Build history of the part. All positions in model axes, mm. A direction names the side the tool comes from. Give positions to 0.01 mm unless a question says otherwise; leave off trailing zeros. Write each loop counter-clockwise with the first axis right and the second up, starting at its lowest first coordinate (ties: lowest second). Pieces come first, ordered by that corner, then holes. Notation, with made-up numbers: (8.25, -11.5) -> (37.25, -11.5) arc R32 ccw to (37.25, 24.5) -> close; hole circle Ø10 at (73.25, 50.5). An arc over 180 degrees is marked (long way). Put each result on its own line as item: value.
from build123d import *

# Parameters (mm, degrees)
BOSS_EXTRUDE1_DEPTH     = 8
BOSS_EXTRUDE2_DEPTH     = 8
SKETCH4_W               = 36.000000000000064
SKETCH4_H               = 30.000000000000057
BOSS_EXTRUDE3_DEPTH     = 8
SKETCH5_R               = 7.000000000000002
SKETCH5_R_2             = 5.000000000000002
BOSS_EXTRUDE4_DEPTH     = 10
CHAMFER1_SIZE           = 3
CUT_EXTRUDE1_REACH      = 260.278
CUT_EXTRUDE2_DEPTH      = 254.2099380250209
SKETCH8_W               = 17.000000000000007
SKETCH8_H               = 20.000000000000043
BOSS_EXTRUDE5_DEPTH     = 7
CUT_EXTRUDE3_DEPTH      = 0.75
CUT_EXTRUDE4_DEPTH      = 0.75
CUT_EXTRUDE5_DEPTH      = 254.2099381566107
CUT_EXTRUDE5_DEPTH_BACK = 254.2099381566107
CUT_EXTRUDE6_DEPTH      = 3
SKETCH14_W              = 9.999999998633207
SKETCH14_H              = 30.000000000000057
CUT_EXTRUDE7_DEPTH      = 3
CUT_EXTRUDE8_START      = -33
CUT_EXTRUDE8_DEPTH      = 30
SKETCH16_W              = 67.2347482813901
SKETCH16_H              = 36.897117956044724
CUT_EXTRUDE9_DEPTH      = 28.75


with BuildPart() as part:
    # Sketch2 → Boss-Extrude1 (new body)
    with BuildSketch(Plane.XY.offset(-8.000000000000261)):
        with BuildLine():
            Line((-25.76918534335193, 245.18029985394168), (-54.787386755608914, 245.18029985394168))
            Line((-54.787386755608914, 245.18029985394168), (-54.787386755608914, 215.18029985394165))
            Line((-54.787386755608914, 215.18029985394165), (-25.76918534335193, 215.18029985394165))
            ThreePointArc((-25.76918534335193, 215.18029985394165), (-10.7691853433519, 230.18029985394168), (-25.76918534335193, 245.18029985394168))
        make_face()
    extrude(amount=BOSS_EXTRUDE1_DEPTH)



with BuildPart() as body_2:
    # Sketch3 → Boss-Extrude2 (new body)
    with BuildSketch(Plane(origin=(4.616e-14, 1.89e-15, -28.000000000000256), x_dir=(-1, 0, -1.65e-15), z_dir=(1.65e-15, 7e-17, -1))):
        with BuildLine():
            Line((25.769185343351936, 215.18029985394165), (54.78738675560893, 215.18029985394165))
            Line((54.78738675560893, 215.18029985394165), (54.78738675560893, 245.18029985394168))
            Line((54.78738675560893, 245.18029985394168), (25.76918534335194, 245.18029985394168))
            ThreePointArc((25.76918534335194, 245.18029985394168), (10.769185343351939, 230.18029985394168), (25.769185343351936, 215.18029985394165))
        make_face()
    extrude(amount=BOSS_EXTRUDE2_DEPTH)


with BuildPart() as part_1:
    add(part.part)

    add(body_2.part)  # Boss-Extrude3 merges body 2
    # Sketch4 → Boss-Extrude3 (add)
    with BuildSketch(Plane.ZY.offset(54.787386755608914)):
        with Locations((-18.000000000000345, 230.18029985394168)):
            Rectangle(SKETCH4_W, SKETCH4_H)
    extrude(amount=BOSS_EXTRUDE3_DEPTH)

    # Sketch5 → Boss-Extrude4 (add)
    with BuildSketch(Plane.ZY.offset(62.78738675560891)):
        with Locations((-18.00000000000032, 230.18029985394168)):
            Circle(SKETCH5_R)
        with Locations((-18.00000000000032, 230.18029985394168)):
            Circle(SKETCH5_R_2, mode=Mode.SUBTRACT)
    extrude(amount=BOSS_EXTRUDE4_DEPTH)

    # Chamfer1
    chamfer1_edges = [part_1.edges().sort_by_distance(p)[0] for p in [
        (-62.78738675560891, 230.18029985394168, -25.00000000000032),
    ]]
    chamfer(chamfer1_edges, length=CHAMFER1_SIZE)

    # Cut-Extrude1: up to this face of the body (flat: up to its plane)
    cut_extrude1_end = Plane(part_1.part.faces().sort_by_distance((-38.272954764, 230.180299854, 0))[0])
    # Sketch6 → Cut-Extrude1 (cut, up to the picked face)
    with BuildSketch(Plane(origin=(0, 0, -36.00000000000038), x_dir=(-1, 0, 0), z_dir=(0, 0, -1)), mode=Mode.PRIVATE) as cut_extrude1_sk1:
        with BuildLine():
            Line((23.93206803626449, 232.05529985394165), (27.606302650439275, 232.05529985394165))
            ThreePointArc((27.606302650439275, 232.05529985394165), (28.39418534335189, 230.18029985394165), (27.606302650439247, 228.30529985394165))
            Line((27.606302650439247, 228.30529985394165), (23.932068036264518, 228.30529985394165))
            ThreePointArc((23.932068036264518, 228.30529985394165), (23.144185343351896, 230.18029985394165), (23.93206803626449, 232.05529985394165))
        make_face()
    cut_extrude1_tool1 = split(extrude(cut_extrude1_sk1.sketch, amount=-CUT_EXTRUDE1_REACH, mode=Mode.PRIVATE), bisect_by=cut_extrude1_end, keep=Keep.BOTH, mode=Mode.PRIVATE)
    add(cut_extrude1_tool1.solids().sort_by(Axis((-25.769185, 230.1803, -36), (0, 0, 1)))[0], mode=Mode.SUBTRACT)

    # Sketch7 → Cut-Extrude2 (cut, through all)
    with BuildSketch(Plane.ZY.offset(62.78738675560891)):
        with BuildLine():
            Line((-3.1052e-13, 215.18029985394165), (-3.1052e-13, 218.18029985394165))
            ThreePointArc((-3.1052e-13, 218.18029985394165), (-0.878679656440668, 216.05897951038202), (-3.0000000000003104, 215.18029985394165))
            Line((-3.0000000000003104, 215.18029985394165), (-3.1052e-13, 215.18029985394165))
        make_face()
        with BuildLine():
            Line((-36.000000000000384, 215.18029985394165), (-33.00000000000038, 215.18029985394165))
            ThreePointArc((-33.00000000000038, 215.18029985394165), (-35.12132034356002, 216.058979510382), (-36.000000000000384, 218.18029985394165))
            Line((-36.000000000000384, 218.18029985394165), (-36.000000000000384, 215.18029985394165))
        make_face()
    extrude(amount=-CUT_EXTRUDE2_DEPTH, mode=Mode.SUBTRACT)

    # Sketch8 → Boss-Extrude5 (add)
    with BuildSketch(Plane.XZ.offset(-215.18029985394165)):
        with Locations((-48.28738675560892, -18.000000000000284)):
            Rectangle(SKETCH8_W, SKETCH8_H)
    extrude(amount=-BOSS_EXTRUDE5_DEPTH)

    # Sketch10 → Cut-Extrude3 (cut)
    with BuildSketch(Plane.XY.offset(-28.000000000000256)):
        with BuildLine():
            Line((-54.78738675560893, 222.18029985394168), (-39.78738675560896, 222.18029985394168))
            Line((-39.78738675560896, 222.18029985394168), (-39.78738675560896, 215.18029985394165))
            Line((-39.78738675560896, 215.18029985394165), (-25.769185343351936, 215.18029985394165))
            ThreePointArc((-25.769185343351936, 215.18029985394165), (-10.76918534335191, 230.18029985394168), (-25.76918534335194, 245.18029985394168))
            Line((-25.76918534335194, 245.18029985394168), (-54.78738675560893, 245.18029985394168))
            Line((-54.78738675560893, 245.18029985394168), (-54.78738675560893, 222.18029985394168))
        make_face()
    extrude(amount=-CUT_EXTRUDE3_DEPTH, mode=Mode.SUBTRACT)

    # Sketch11 → Cut-Extrude4 (cut)
    with BuildSketch(Plane(origin=(0, 0, -8.000000000000261), x_dir=(-1, 0, 0), z_dir=(0, 0, -1))):
        with BuildLine():
            Line((25.76918534335193, 215.18029985394165), (39.787386755608914, 215.18029985394165))
            Line((39.787386755608914, 215.18029985394165), (39.787386755608914, 222.18029985394168))
            Line((39.787386755608914, 222.18029985394168), (54.787386755608914, 222.18029985394168))
            Line((54.787386755608914, 222.18029985394168), (54.787386755608914, 245.18029985394168))
            Line((54.787386755608914, 245.18029985394168), (25.76918534335193, 245.18029985394168))
            ThreePointArc((25.76918534335193, 245.18029985394168), (10.769185343351928, 230.18029985394168), (25.76918534335193, 215.18029985394165))
        make_face()
    extrude(amount=-CUT_EXTRUDE4_DEPTH, mode=Mode.SUBTRACT)

    # Sketch12 → Cut-Extrude5 (cut, two sides: drawn at the far end of the back side and taken through both)
    with BuildSketch(Plane.ZY.offset(62.78738675560891).offset(-CUT_EXTRUDE5_DEPTH_BACK)):
        with BuildLine():
            Line((-23.750000000000245, 242.68029985394168), (-12.25000000000027, 242.68029985394168))
            ThreePointArc((-12.25000000000027, 242.68029985394168), (-11.542893218813717, 242.38740663512823), (-11.250000000000261, 241.68029985394168))
            Line((-11.250000000000261, 241.68029985394168), (-11.250000000000261, 239.18029985394168))
            ThreePointArc((-11.250000000000261, 239.18029985394168), (-11.542893218813717, 238.47319307275512), (-12.25000000000027, 238.18029985394168))
            Line((-12.25000000000027, 238.18029985394168), (-23.750000000000245, 238.18029985394168))
            ThreePointArc((-23.750000000000245, 238.18029985394168), (-24.4571067811868, 238.47319307275512), (-24.750000000000256, 239.18029985394168))
            Line((-24.750000000000256, 239.18029985394168), (-24.750000000000256, 241.68029985394168))
            ThreePointArc((-24.750000000000256, 241.68029985394168), (-24.4571067811868, 242.38740663512823), (-23.750000000000245, 242.68029985394168))
        make_face()
    extrude(amount=CUT_EXTRUDE5_DEPTH + CUT_EXTRUDE5_DEPTH_BACK, mode=Mode.SUBTRACT)

    # Sketch13 → Cut-Extrude6 (cut)
    with BuildSketch(Plane(origin=(0, 0, -36.00000000000038), x_dir=(-1, 0, 0), z_dir=(0, 0, -1))):
        Polygon((52.78738675697571, 245.1803259806636), (65.22032452313796, 245.1803259806636), (65.22032452313796, 215.18029985394165), (52.787386756975714, 215.18029985394165), align=None)
    extrude(amount=-CUT_EXTRUDE6_DEPTH, mode=Mode.SUBTRACT)

    # Sketch14 → Cut-Extrude7 (cut)
    with BuildSketch(Plane.XY):
        with Locations((-57.78738675629231, 230.18029985394168)):
            Rectangle(SKETCH14_W, SKETCH14_H)
    extrude(amount=-CUT_EXTRUDE7_DEPTH, mode=Mode.SUBTRACT)

    # Sketch15 → Cut-Extrude8 (cut)
    with BuildSketch(Plane.XY.offset(CUT_EXTRUDE8_START)):
        with BuildLine():
            add(Edge.make_bspline(
                [(-58.787343120375006, 241.68025514760154), (-61.78734312026629, 241.68025514726713), (-61.78734312015468, 238.68025514738127), (-58.7873431202634, 238.68025514771568), (-55.78734312037213, 238.6802551480501), (-55.78734312048373, 241.68025514793592), (-58.787343120375006, 241.68025514760154)],
                knots=[0, 0, 0, 0, 0.5, 0.5, 0.5, 1, 1, 1, 1], degree=3, weights=[1, 0.33333333333333337, 0.33333333333333337, 1, 0.33333333333333337, 0.33333333333333337, 1]))
        make_face()
        with BuildLine():
            add(Edge.make_bspline(
                [(-58.787343119686746, 223.17998583120436), (-61.78734311957803, 223.17998583086998), (-61.78734311946642, 220.17998583098415), (-58.787343119575134, 220.1799858313185), (-55.78734311968384, 220.1799858316529), (-55.78734311979546, 223.17998583153874), (-58.787343119686746, 223.17998583120436)],
                knots=[0, 0, 0, 0, 0.5, 0.5, 0.5, 1, 1, 1, 1], degree=3, weights=[1, 0.33333333333333337, 0.33333333333333337, 1, 0.33333333333333337, 0.33333333333333337, 1]))
        make_face()
    extrude(amount=CUT_EXTRUDE8_DEPTH, mode=Mode.SUBTRACT)

    # Sketch16 → Cut-Extrude9 (cut)
    with BuildSketch(Plane.XY):
        with Locations((-42.47434442630761, 229.60312045940518)):
            Rectangle(SKETCH16_W, SKETCH16_H)
    extrude(amount=-CUT_EXTRUDE9_DEPTH, mode=Mode.SUBTRACT)


solid = part_1.part
1) Wall check: L1, parallel to X at y = 230, z = -29.25; L2, parallel to X at y = 240, z = -30.25; L3, parallel to Z at x = -53.5, y = 233. Give the ranges that are in metal, low to high.
Filled sheet:
L1: -62.79 to -28.39, -23.15 to -10.77
L2: -62.79 to -60.28, -57.3 to -14.43
L3: -33 to -28.75
2) Tool access for faces 4 (the flat face through (-31, 231, -36)), 5 (the flat face through (-26, 232.055, -32)), 6 (the flat face through (-58, 230, -33)): list every direction of +Z, -Z, +X, -X, +Y, -Y with a clear straight run to the whole face (end or side of a thin tool).
Filled sheet:
face 4: -Z, +X, -X, +Y, -Y
face 5: +Z, -Z
face 6: -Z, -X, +Y, -Y
3) Pin check, flat tips, straight feed: pin 1 (3 mm diameter, centred on y = 221, z = -31.5, fed in from +X); pin 2 (5 mm diameter, centred on x = -59.5, y = 223.5, fed in from -Z); pin 3 (1.5 mm diameter, centred on y = 229.5, z = -33.5, fed in from +X); pin 4 (0.9 mm diameter, centred on y = 232, z = -34, fed in from -X). Stop position of each tip, or through.
Filled sheet:
pin 1: x = -12.88
pin 2: z = -33
pin 3: x = -10.77
pin 4: x = -52.79
4) Slice it at A-A (z = -34.25). Write the cut outline in (x, y) (3 decimals), plus the area to 3 significant figures.
Filled sheet:
outline: (-52.787, 215.453) -> (-22.921, 215.453) arc R15 ccw to (-25.769, 245.18) -> (-52.787, 245.18) -> close; hole (-27.606, 228.305) -> (-23.932, 228.305) arc R2.625 ccw to (-23.932, 232.055) -> (-27.606, 232.055) arc R2.625 ccw to start
area: 1,140 mm2
5) Slice it at C-C (z = -31.75). Give the number of separate pieces and of enclosed holes in the cut face, plus the area to 3 significant figures.
Filled sheet:
separate pieces: 1
enclosed holes: 3
area: 1,430 mm2
6) Pull direction Y, two halves, no side cores. Call faces 1 (the cylindrical face through (-28.394, 230.21, -32.426)), 2 (the cylindrical face through (-10.773, 230.51, -32.324)), 3 (the flat face through (-52.787, 230, -35)): released by +Y, released by -Y, zero draft, split by the parting line, or undercut.
Filled sheet:
face 1: undercut
face 2: split by the parting line
face 3: zero draft
7) Slice it at B-B (y = 234). Write the cut outline in (x, z), plus the area to 3 significant figures.
Filled sheet:
outline: (-62.79, -33) -> (-52.79, -33) -> (-52.79, -36) -> (-11.26, -36) -> (-11.26, -28.75) -> (-62.79, -28.75) -> close
area: 344 mm2
8) Slice it at D-D (y = 227). Write the cut outline in (x, z).
Filled sheet:
outline: (-62.79, -33) -> (-52.79, -33) -> (-52.79, -36) -> (-11.11, -36) -> (-11.11, -28.75) -> (-62.79, -28.75) -> close
